```python
from build123d import *

# Parameters (mm, degrees)
SKETCH1_R                 = 6
BOSS_EXTRUDE1_DEPTH       = 5
CUT_EXTRUDE1_DEPTH        = 3
SKETCH3_R                 = 4.075
BOSS_EXTRUDE2_DEPTH       = 7
SKETCH4_R                 = 5.7
BOSS_EXTRUDE3_DEPTH       = 18.5
F_1_0MM_DOWEL_HOLE1_D     = 3
F_1_0MM_DOWEL_HOLE1_DEPTH = 30.5
F_1_0MM_DOWEL_HOLE1_TIP   = 0.901290929


with BuildPart() as part:
    # Sketch1 → Boss-Extrude1 (new body)
    with BuildSketch(Plane(origin=(0, 0, 0), x_dir=(1, 0, 0), z_dir=(0, 1, 0))):
        with Locations(Location((0, 0, 0), (0, 0, 270))):
            Circle(SKETCH1_R)
    extrude(amount=BOSS_EXTRUDE1_DEPTH)

    # Sketch2 → Cut-Extrude1 (cut)
    with BuildSketch(Plane.XZ):
        Polygon((3.233161507, 0), (1.616580754, 2.8), (-1.616580754, 2.8), (-3.233161507, 0), (-1.616580754, -2.8), (1.616580754, -2.8), align=None)
    extrude(amount=-CUT_EXTRUDE1_DEPTH, mode=Mode.SUBTRACT)

    # Sketch3 → Boss-Extrude2 (add)
    with BuildSketch(Plane(origin=(0, 5, 0), x_dir=(1, 0, 0), z_dir=(0, 1, 0))):
        with Locations(Location((0, 0, 0), (0, 0, 270))):
            Circle(SKETCH3_R)
    extrude(amount=BOSS_EXTRUDE2_DEPTH)

    # Sketch4 → Boss-Extrude3 (add)
    with BuildSketch(Plane(origin=(0, 12, 0), x_dir=(1, 0, 0), z_dir=(0, 1, 0))):
        with Locations(Location((0, 0, 0), (0, 0, 270))):
            Circle(SKETCH4_R)
    extrude(amount=BOSS_EXTRUDE3_DEPTH)

    # Ø1.0mm Dowel Hole1
    with Locations(Plane(origin=(0, 30.5, 0), x_dir=(1, 0, 0), z_dir=(0, 1, 0))):
        with Locations((0, 0)):
            Hole(F_1_0MM_DOWEL_HOLE1_D / 2, depth=F_1_0MM_DOWEL_HOLE1_DEPTH)
            with Locations((0, 0, -(F_1_0MM_DOWEL_HOLE1_DEPTH + F_1_0MM_DOWEL_HOLE1_TIP / 2))):  # 118° drill point
                Cone(0, F_1_0MM_DOWEL_HOLE1_D / 2, F_1_0MM_DOWEL_HOLE1_TIP, mode=Mode.SUBTRACT)


solid = part.part
```
Model file for the job. Use its own axes, mm. A direction names the side the tool comes from. Coordinates: 2 decimals unless noted, no trailing zeros. Order: outer loops, then holes, each group sorted by start corner. A loop starts at its lowest first (then second) coordinate and runs counter-clockwise, first axis right, second up. Notation, with made-up numbers: (60.25, 9) -> (117.25, 9) arc R14 ccw to (117.25, 32) -> close; hole circle Ø8 at (35, 88.5). An arc over 180 degrees is marked (long way). Answer as a JSON object with one key per item and string values. Group by question number.
1) Cut at B-B, the plane z = 5.25. Write the cut outline in (x, y).
2) Drill centre lines: L1, parallel to Y at x = 0.5, z = 5; L2, parallel to Y at x = 5.5, z = -2; L3, parallel to X at y = 23, z = 1.25. Where is each one in solid material? Low to high.
3) Cut at C-C, the plane y = 7. Write the cut outline in (x, z) (3 decimals).
4) Pull direction Z, two halves, no side cores. Call faces 6 (the face through (-1.2, 30.5, 1.2)), 7 (the face through (2.414, 1.479, -1.42)), 8 (the face through (-2.48, 8.451, -3.234)): +Z half, -Z half, draft (parallel to the pull), parting line (faces both ways), or undercut.
5) Cut at A-A, the plane x = 0. Write the cut outline in (y, z) (3 decimals).
6) Which spindle directions (+Z, -Z, +X, -X, +Y, -Y) get a long thin tool onto all of the face, cutting with end or side? Do faces 1 (the face through (-3.5, 21.1, -4.5)), 2 (the face through (2.436, 1.479, 1.38)), 3 (the face through (-4, 12, 2)), 4 (the face through (-3, 0, 1)), 5 (the face through (1.5, 16.56, -0.07)). Say none if no direction does.
7) Cut at D-D, the plane z = -3.75. Write the cut outline in (x, y).
8) Flat gauge pins, fed straight in: pin 1 (5 mm diameter, centred on x = 5, y = 24.5, fed in from +Z); pin 2 (1.5 mm diameter, centred on y = 19, z = -3, fed in from -X). Where does each tip first touch, or does it go through?
Check values:
{
 "1": {"outline": "(-2.9, 0) -> (2.9, 0) -> (2.9, 5) -> (-2.9, 5) -> close; (-2.22, 12) -> (2.22, 12) -> (2.22, 30.5) -> (-2.22, 30.5) -> close"},
 "2": {"L1": "y = 0 to 5, 12 to 30.5", "L2": "y = 0 to 5", "L3": "x = -5.56 to -0.83, 0.83 to 5.56"},
 "3": {"outline": "circle Ø8.15 at (0, 0); hole circle Ø3 at (0, 0)"},
 "4": {"face 6": "draft", "face 7": "undercut", "face 8": "parting line"},
 "5": {"outline": "(0, -6) -> (5, -6) -> (5, -4.075) -> (12, -4.075) -> (12, -5.7) -> (30.5, -5.7) -> (30.5, -1.5) -> (3, -1.5) -> (3, -2.8) -> (0, -2.8) -> close; (0, 2.8) -> (3, 2.8) -> (3, 1.5) -> (30.5, 1.5) -> (30.5, 5.7) -> (12, 5.7) -> (12, 4.075) -> (5, 4.075) -> (5, 6) -> (0, 6) -> close"},
 "6": {"face 1": "+Y", "face 2": "-Y", "face 3": "none", "face 4": "+Z, -Z, +X, -X, -Y", "face 5": "+Y, -Y"},
 "7": {"outline": "(-4.68, 0) -> (4.68, 0) -> (4.68, 5) -> (1.59, 5) -> (1.59, 12) -> (4.29, 12) -> (4.29, 30.5) -> (-4.29, 30.5) -> (-4.29, 12) -> (-1.59, 12) -> (-1.59, 5) -> (-4.68, 5) -> close"},
 "8": {"pin 1": "stops at z = 5.12", "pin 2": "stops at x = -5.24"}
}
